Could you check a few things on this model? Use its own coordinates, in mm. A direction names the side the tool comes from. Coordinates: 2 decimals unless noted, no trailing zeros. Loops run counter-clockwise (first coordinate to the right, second up) from the corner with the lowest first, then second, coordinate; pieces in that order, holes last.
from build123d import *

# Parameters (mm, degrees)
SKETCH1_W           = 66
SKETCH1_H           = 143
SKETCH1_R           = 16
SKETCH1_R_2         = 5.2
SKETCH1_R_3         = 11.3
SKETCH1_R_4         = 1.7
BOSS_EXTRUDE1_DEPTH = 12
SKETCH3_R           = 18.6
SKETCH3_W           = 40.2
SKETCH3_H           = 40.2
CUT_EXTRUDE1_DEPTH  = 8
SKETCH4_R           = 23.6
CUT_EXTRUDE2_DEPTH  = 6
SKETCH5_R           = 6
BOSS_EXTRUDE2_DEPTH = 12
SKETCH5_3_R         = 3
CUT_EXTRUDE3_DEPTH  = 120.82069938
FILLET1_R           = 30
VERRUNDUNG1_R       = 10


with BuildPart() as part:
    # Sketch1 → Boss-Extrude1 (new body)
    with BuildSketch(Plane.XY):
        with Locations((0, 41.5)):
            Rectangle(SKETCH1_W, SKETCH1_H)
        Circle(SKETCH1_R, mode=Mode.SUBTRACT)
        with Locations((0, 50)):
            Circle(SKETCH1_R_2, mode=Mode.SUBTRACT)
        with Locations((0, 92)):
            Circle(SKETCH1_R_3, mode=Mode.SUBTRACT)
        with Locations((-9.9, 101.9)):
            Circle(SKETCH1_R_4, mode=Mode.SUBTRACT)
        with Locations((9.9, 101.9)):
            Circle(SKETCH1_R_4, mode=Mode.SUBTRACT)
        with Locations((9.9, 82.1)):
            Circle(SKETCH1_R_4, mode=Mode.SUBTRACT)
        with Locations((-9.9, 82.1)):
            Circle(SKETCH1_R_4, mode=Mode.SUBTRACT)
    extrude(amount=BOSS_EXTRUDE1_DEPTH)

    # Sketch3 → Cut-Extrude1 (cut)
    with BuildSketch(Plane.XY.offset(12)):
        with Locations((0, 92)):
            Circle(SKETCH3_R)
        with Locations((0, 50)):
            Rectangle(SKETCH3_W, SKETCH3_H)
    extrude(amount=-CUT_EXTRUDE1_DEPTH, mode=Mode.SUBTRACT)

    # Sketch4 → Cut-Extrude2 (cut)
    with BuildSketch(Plane.XY.offset(12)):
        Circle(SKETCH4_R)
    extrude(amount=-CUT_EXTRUDE2_DEPTH, mode=Mode.SUBTRACT)

    # Sketch5 → Boss-Extrude2 (add)
    with BuildSketch(Plane.XY):
        with Locations((-32, 0)):
            Circle(SKETCH5_R)
        with Locations((32, 0)):
            Circle(SKETCH5_R)
    extrude(amount=BOSS_EXTRUDE2_DEPTH)

    # Sketch5<3> → Cut-Extrude3 (cut, through all)
    with BuildSketch(Plane.XY):
        with Locations((32, 0)):
            Circle(SKETCH5_3_R)
        with Locations((-32, 0)):
            Circle(SKETCH5_3_R)
    extrude(amount=CUT_EXTRUDE3_DEPTH, mode=Mode.SUBTRACT)

    # Fillet1
    # the kernel refuses this fillet: 30 mm, written as the material it takes off along each edge
    with BuildSketch(Plane(origin=(-33, 113, -75), x_dir=(1, 0, 0), z_dir=(0, 0, 1))) as fillet1_piece_1:
        with BuildLine():
            CenterArc((FILLET1_R, -FILLET1_R), FILLET1_R, 90, 90)
            Line((0, -FILLET1_R), (-FILLET1_R * 0.02, -FILLET1_R))
            Line((-FILLET1_R * 0.02, -FILLET1_R), (-FILLET1_R * 0.02, FILLET1_R * 0.02))
            Line((-FILLET1_R * 0.02, FILLET1_R * 0.02), (FILLET1_R, FILLET1_R * 0.02))
            Line((FILLET1_R, FILLET1_R * 0.02), (FILLET1_R, 0))
        make_face()
    extrude(amount=162, mode=Mode.SUBTRACT)
    with BuildSketch(Plane(origin=(33, 113, -75), x_dir=(-1, 0, 0), z_dir=(0, 0, 1))) as fillet1_piece_2:
        with BuildLine():
            CenterArc((FILLET1_R, FILLET1_R), FILLET1_R, 180, 90)
            Line((0, FILLET1_R), (-FILLET1_R * 0.02, FILLET1_R))
            Line((-FILLET1_R * 0.02, FILLET1_R), (-FILLET1_R * 0.02, -FILLET1_R * 0.02))
            Line((-FILLET1_R * 0.02, -FILLET1_R * 0.02), (FILLET1_R, -FILLET1_R * 0.02))
            Line((FILLET1_R, -FILLET1_R * 0.02), (FILLET1_R, 0))
        make_face()
    extrude(amount=162, mode=Mode.SUBTRACT)
    with BuildSketch(Plane(origin=(33, -30, -73.527205849), x_dir=(-1, 0, 0), z_dir=(0, 0, 1))) as fillet1_piece_3:
        with BuildLine():
            CenterArc((29.41088234, -30), FILLET1_R, 90, 78.626574363)
            Line((0, -24.083920217), (-0.588217647, -23.965598621))
            ThreePointArc((-0.588217647, -23.965598621), (-0.6, -12.041960108), (-0.6, 0))
            Line((-0.6, 0), (0, 0.6))
            Line((0, 0.6), (29.41088234, 0.6))
            Line((29.41088234, 0.6), (29.41088234, 0))
        make_face()
    extrude(amount=159.054411699, mode=Mode.SUBTRACT)
    with BuildSketch(Plane(origin=(-33, -30, -73.527205849), x_dir=(0, 1, 0), z_dir=(0, 0, 1))) as fillet1_piece_4:
        with BuildLine():
            CenterArc((30, -29.41088234), FILLET1_R, 101.373425637, 78.626574363)
            Line((0, -29.41088234), (-0.6, -29.41088234))
            Line((-0.6, -29.41088234), (-0.6, 0))
            Line((-0.6, 0), (0, 0.6))
            ThreePointArc((0, 0.6), (12.041960108, 0.6), (23.965598621, 0.588217647))
            Line((23.965598621, 0.588217647), (24.083920217, 0))
        make_face()
    extrude(amount=159.054411699, mode=Mode.SUBTRACT)

    # Verrundung1
    verrundung1_edges = [part.edges().sort_by_distance(p)[0] for p in [
        (-33, 5.916079783, 6),
        (-33, -5.916079783, 6),
        (33, -5.916079783, 6),
        (33, 5.916079783, 6),
    ]]
    fillet(verrundung1_edges, radius=VERRUNDUNG1_R)


solid = part.part
1) Imagine slicing it at B-B on x = 9.9. State how many separate pieces and enclosed holes the cut face has, plus the area to 3 significant figures.
2) We'd pull the mould along X, two halves only. Please class faces 4 (the cylindrical face through (38, 0, 6)), 5 (the cylindrical face through (-38, 0, 6)), 6 (the flat face through (0, 29.9, 8)): released by +X, released by -X, zero draft, split by the parting line, or undercut.
3) If I drill on L1, parallel to Y at x = 0, z = 7.4; L2, parallel to Y at x = -0.5, z = 4.75; L3, parallel to X at y = 70, z = 3, over which ranges is the centre line in solid material (lowest first)?
4) Will these pins go through, and if not, where does the flat tip stop? pin 1 (3 mm diameter, centred on x = 5.5, y = 84.5, fed in from +Z); pin 2 (6.5 mm diameter, centred on x = -10, z = 9.5, fed in from +Y); pin 3 (5.5 mm diameter, centred on x = -9.9, y = 82.1, fed in from +Z); pin 4 (6.5 mm diameter, centred on x = 9.5, z = 7.5, fed in from -Y).
5) Imagine slicing it at C-C on x = 0. List the corners of the cut face in (y, z) for me, plus the area to 3 significant figures.
6) For faces 1 (the flat face through (-33, 47, 6)), 2 (the flat face through (33, 47, 6)), 3 (the flat face through (12, 92, 4)), which set-ups out of +Z, -Z, +X, -X, +Y, -Y let a thin tool reach every point of the face, with its end or its side?
7) Imagine slicing it at D-D on y = 92. List the corners of the cut face in (x, z) for me, plus the area to 3 significant figures.
8) Imagine slicing it at A-A on y = 0. List the corners of the cut face in (x, z) for me, plus the area to 3 significant figures.
Solved:
1. separate pieces: 5
1. enclosed holes: 0
1. area: 646 mm2
2. face 4: released by +X
2. face 5: released by -X
2. face 6: undercut
3. L1: y = -30 to -23.6, 23.6 to 29.9, 70.1 to 73.4, 110.6 to 113
3. L2: y = -30 to -15.99, 15.99 to 29.9, 70.1 to 73.41, 110.59 to 113
3. L3: x = -33 to 33
4. pin 1: passes through
4. pin 2: stops at y = 112.76
4. pin 3: stops at z = 4
4. pin 4: stops at y = -29.88
5. outline: (-30, 0) - (-16, 0) - (-16, 6) - (-23.6, 6) - (-23.6, 12) - (-30, 12) - close; (16, 0) - (44.8, 0) - (44.8, 4) - (29.9, 4) - (29.9, 12) - (23.6, 12) - (23.6, 6) - (16, 6) - close; (55.2, 0) - (80.7, 0) - (80.7, 4) - (73.4, 4) - (73.4, 12) - (70.1, 12) - (70.1, 4) - (55.2, 4) - close; (103.3, 0) - (113, 0) - (113, 12) - (110.6, 12) - (110.6, 4) - (103.3, 4) - close
5. area: 490 mm2
6. face 1: +Z, -Z, -X, +Y
6. face 2: +Z, -Z, +X, +Y
6. face 3: +Z
7. outline: (-31.62, 0) - (-11.3, 0) - (-11.3, 4) - (-18.6, 4) - (-18.6, 12) - (-31.62, 12) - close; (11.3, 0) - (31.62, 0) - (31.62, 12) - (18.6, 12) - (18.6, 4) - (11.3, 4) - close
7. area: 371 mm2
8. outline: (-38, 0) - (-35, 0) - (-35, 12) - (-38, 12) - close; (-29, 0) - (-16, 0) - (-16, 6) - (-23.6, 6) - (-23.6, 12) - (-29, 12) - close; (16, 0) - (29, 0) - (29, 12) - (23.6, 12) - (23.6, 6) - (16, 6) - close; (35, 0) - (38, 0) - (38, 12) - (35, 12) - close
8. area: 293 mm2
